Job drawing, mm, ordinate dimensions from the low corner. One solid piece. Give positions to 0.01 mm unless a question says otherwise; leave off trailing zeros. Loops run counter-clockwise (first coordinate to the right, second up) from the corner with the lowest first, then second, coordinate; pieces in that order, holes last. Notation, with made-up numbers: (52.25, -34.75) -> (74.25, -34.75) arc R15 ccw to (74.25, -11.75) -> close; hole circle Ø6 at (81.25, 45.25). An arc over 180 degrees is marked (long way). Answer as a JSON object with one key per item and string values. Group by question number.
Q1. Drop flat-ended pins along their axis: pin 1 (3 mm diameter, centred on x = 357.5, z = 14.5, fed in from +Y); pin 2 (1 mm diameter, centred on y = 169.5, z = 8, fed in from +X); pin 3 (8 mm diameter, centred on y = 221.5, z = 7, fed in from -X). Give the stop position or say it passes through.
Q2. Wall check: probe 1 along Y at (x, z) = (573.5, 6.75); probe 2 along X at (y, z) = (190, 4); probe 3 along Y at (x, z) = (234.5, 7.5). Give the ranges that are in metal, low to high. Write a range as from..to.
Q3. Band-saw the part on C-C, the plane y = 21. Write the cut outline in (x, z).
Q4. Band-saw the part on B-B, the plane z = 10.25. Write the cut outline in (x, y), plus the area to 3 significant figures.
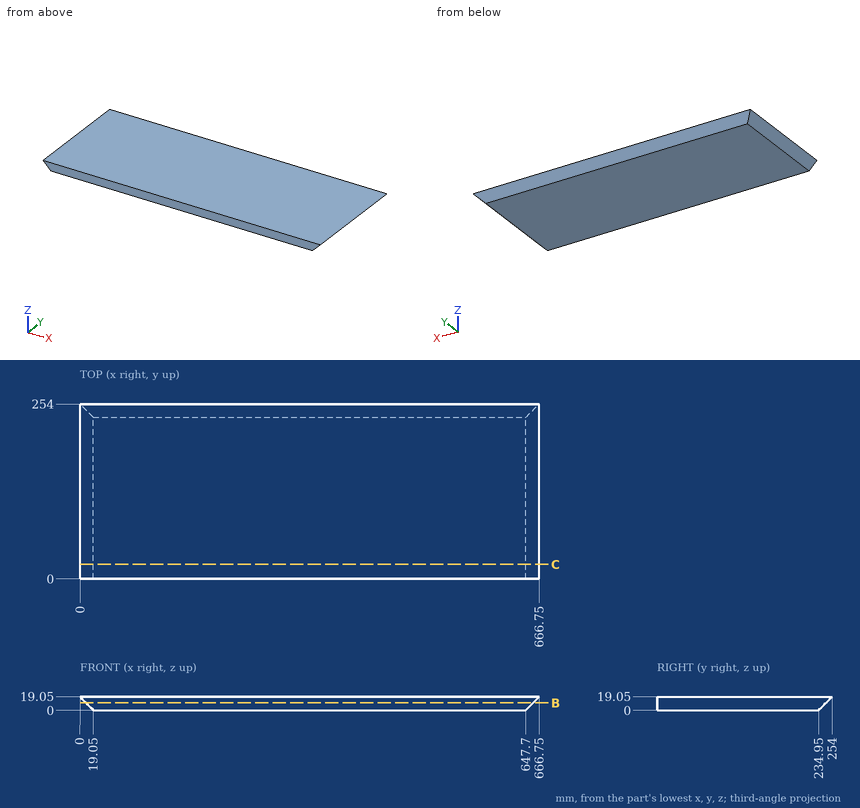
Worked answers:
{
 "1": {"pin 1": "y = 250.95", "pin 2": "x = 656.2", "pin 3": "x = 8.05"},
 "2": {"probe 1": "0..241.7", "probe 2": "15.05..651.7", "probe 3": "0..242.45"},
 "3": {"outline": "(0, 19.05) -> (19.05, 0) -> (647.7, 0) -> (666.75, 19.05) -> close"},
 "4": {"outline": "(8.8, 0) -> (657.95, 0) -> (657.95, 245.2) -> (8.8, 245.2) -> close", "area": "159,000 mm2"}
}
